Autodesk Inventor part; units mm, degrees
ref_plane "YZ Plane" through (0, 0, 0) normal (1, 0, 0) x (0, 1, 0)
ref_plane "XZ Plane" through (0, 0, 0) normal (0, 1, 0) x (-1, 0, 0)
ref_plane "XY Plane" through (0, 0, 0) normal (0, 0, 1) x (1, 0, 0)
ref_plane "Work Plane1" through (0, 0, 0) normal (0, 0, 1) x (1, 0, 0)
sketch "Sketch1" plane through (0, 0, 0) normal (0, 0, 1) x (1, 0, 0)
  circle A0 centre (132.5, -74.5) radius 1.45
  circle A1 centre (177, -74.5) radius 1.45
  line L0 (128.75, -70.75) -> (180.75, -70.75)
  line L1 (180.75, -70.75) -> (180.75, -78.25)
  line L2 (180.75, -78.25) -> (128.75, -78.25)
  line L3 (128.75, -78.25) -> (128.75, -70.75)
  circle A2 centre (132.5, -74.5) radius 1.45
  circle A3 centre (177, -74.5) radius 1.45
  point P0 (0, 0)
  dimension "d0" = 3.75
  dimension "d1" = 3.75
  dimension "d2" = 3.75
  dimension "d3" = 3.75
extrude "Extrusion1" add sketch "Sketch1" along normal blind 15
sketch "Sketch2" plane through (0, 0, 15) normal (0, 0, 1) x (1, 0, 0)
  line L0 (128.75, -78.25) -> (180.75, -78.25)
  line L1 (180.75, -78.25) -> (180.75, -70.75)
  line L2 (180.75, -70.75) -> (128.75, -70.75)
  line L3 (128.75, -70.75) -> (128.75, -78.25)
  circle A0 centre (177, -74.5) radius 1.45
  circle A1 centre (132.5, -74.5) radius 1.45
  circle A2 centre (177, -74.5) radius 1.45
  circle A3 centre (132.5, -74.5) radius 1.45
  point P0 (0, 0)
extrude "Extrusion2" add sketch "Sketch2" against normal blind 8 contours A1
sketch "Sketch4" plane through (0, 0, 15) normal (0, 0, 1) x (1, 0, 0)
  circle A0 centre (177, -74.5) radius 1.45
  circle A1 centre (177, -74.5) radius 1.45
  point P0 (0, 0)
extrude "Extrusion3" add sketch "Sketch4" against normal blind 8
sketch "Sketch5" plane through (128.75, -70.75, 0) normal (0, 1, 0) x (1, 0, 0)
  line L0 (52, 0) -> (0, 0)
  line L1 (0, 0) -> (0, -15)
  line L2 (52, -15) -> (0, -15)
  line L3 (52, 0) -> (52, -15)
  line L4 (52, -15) -> (0, -15)
  line L5 (0, -15) -> (0, 0)
  line L6 (0, 0) -> (52, 0)
  line L7 (52, 0) -> (52, -15)
  line L8 (52, -15) -> (0, -15)
  line L9 (27.805, -15) -> (30.495, -15)
  line L10 (30.495, -16) -> (27.805, -16)
  line L11 (30.495, -16) -> (30.495, -15)
  line L12 (27.805, -16) -> (27.805, -15)
  line L13 (0, -15) -> (52, -15)
  line L14 (32.545, -15) -> (52, -7.5)
  line L15 (52, 0) -> (52, -15)
  line L16 (41.9691, -6) -> (34.1871, -9) construction
  line L17 (42.5086, -7.3996) -> (34.7266, -10.3996)
  line L18 (33.6475, -7.6004) -> (41.4295, -4.6004)
  arc A0 (42.5086, -7.3996) -> (41.4295, -4.6004) centre (41.9691, -6) ccw
  arc A1 (33.6475, -7.6004) -> (34.7266, -10.3996) centre (34.1871, -9) ccw
  line L19 (20.0475, -7.6004) -> (27.8295, -4.6004)
  arc A2 (20.0475, -7.6004) -> (21.1266, -10.3996) centre (20.5871, -9) ccw
  line L20 (28.9086, -7.3996) -> (21.1266, -10.3996)
  arc A3 (28.9086, -7.3996) -> (27.8295, -4.6004) centre (28.3691, -6) ccw
  line L21 (-13.6, 0) -> (38.4, 0)
  line L22 (6.4475, -7.6004) -> (14.2295, -4.6004)
  arc A4 (6.4475, -7.6004) -> (7.5266, -10.3996) centre (6.9871, -9) ccw
  line L23 (15.3086, -7.3996) -> (7.5266, -10.3996)
  arc A5 (15.3086, -7.3996) -> (14.2295, -4.6004) centre (14.7691, -6) ccw
  line L24 (-27.2, 0) -> (24.8, 0)
  point P0 (-128.75, 0)
  point P1 (38.0781, -7.5)
  point P2 (52, -7.5)
  point P3 (32.545, -15)
  dimension "d15" = 2.05
  dimension "d21" = 6
  dimension "d22" = 6
  dimension "d23" = 1.5
  dimension "d26" = 13.6
sketch "Sketch6" plane through (0, 0, 15) normal (0, 0, 1) x (1, 0, 0)
  circle A0 centre (132.5, -74.5) radius 1.45
  line L0 (128.75, -78.25) -> (180.75, -78.25)
  line L1 (180.75, -78.25) -> (180.75, -70.75)
  line L2 (180.75, -70.75) -> (128.75, -70.75)
  line L3 (128.75, -70.75) -> (128.75, -78.25)
  circle A1 centre (132.499, -74.9265) radius 1.45
  point P0 (0, 0)
  point P1 (132.5, -74.5)
  dimension "d10" = 2.9
  dimension "d14" = 0.4265
extrude "Extrusion4" cut sketch "Sketch6" against normal blind 7 contours A1 A0 | A0 A1 picked at (132.385, -75.1117) picked at (132.6881, -76.0727)
extrude "Extrusion5" cut sketch "Sketch5" against normal blind 8 contours L3 L2 L14 | L17 A1 L18 A0 | L19 A3 L20 A2 | L22 A5 L23 A4
fillet "Fillet1" radius 1.5 3 edges at (180.75, -74.5, 7.5) (161.295, -74.5, 15) (128.75, -74.5, 15)
sketch "Sketch8" plane through (0, 0, 15) normal (0, 0, 1) x (1, 0, 0)
  circle A0 centre (157.9, -75.0575) radius 1.345
  ellipse E0 centre (158.6032, -73.9122) end of major axis (157.4109, -73.2898) minor radius 1.3427
  point P0 (0, 0)
extrude "Extrusion7" cut sketch "Sketch8" against normal blind 6.5 contours A0 E0 | A0 E0 picked at (158.3944, -74.3129) picked at (159.1018, -73.1783)
properties part number "PCB-LNA_Print_CPY"
The listing builds one solid part. Answer for the finished solid, in the listing's coordinates (mm). A direction names the side the tool comes from. Give positions to 0.01 mm unless a question says otherwise; leave off trailing zeros. Loops run counter-clockwise (first coordinate to the right, second up) from the corner with the lowest first, then second, coordinate; pieces in that order, holes last. Notation, with made-up numbers: (69.5, -30) - (124.5, -30) arc R22 cw to (124.5, -5) - close; hole circle Ø1 at (80, 73). An arc over 180 degrees is marked (long way). Return JSON: item names as keys, results as strings. Group by question number.
1. Given pin 1 Ø0.8 at (x, y) = (159, -74) entering from +Z; pin 2 Ø4.5 at (x, y) = (177, -74.5) entering from +Z; pin 3 Ø1.4 at (x, y) = (132.5, -75) entering from +Z, each flat-ended and moving along its own axis, determine where each tip first touches the part or whether it passes through.
2. Find section C-C (z = 5.75). Write down the section's boundary in (x, y).
3. Straight lines are drawn through the part: line 1 (X direction, y = -74.5, z = 3.75); line 2 (Y direction, x = 177, z = 6); line 3 (X direction, y = -75.75, z = 3.5). For each, find the intervals that lie inside material, in ascending order. Write a range as [from, to].
4. Which of the six approach directions +Z, -Z, +X, -X, +Y, -Y give full straight-line access (tool end or side, diameter ignored) to faces 5 (the cylindrical face through (133.839, -73.945, 3.451)), 6 (the flat face through (166.234, -74.448, 6.121)), 7 (the flat face through (154, -70.75, 9)), 8 (the flat face through (132, -75, 8)), 9 (the cylindrical face through (180.5, -74.6, 7.3))?
5. Find section D-D (x = 155). Write down the section's boundary in (y, z), then the cut area to 3 significant figures.
6. Find section B-B (z = 2.5). Write down the section's boundary in (x, y).
7. Find section A-A (y = -71.5). Write down the section's boundary in (x, z), then the cut area to 3 significant figures.
8. Determine the mould class of faces 1 (the cylindrical face through (178.339, -73.945, 3.451)), 2 (the cylindrical face through (147.926, -74.448, 9.509)), 3 (the flat face through (159, -74, 8.5)), 4 (the flat face through (139.034, -74.448, 6.121)) for opening direction Z: pulls with the +Z half, pulls with the -Z half, needs draft (parallel to the pull), parting line crosses it, or undercut.
Verdict:
{
 "1": {"pin 1": "stops at z = 8.5", "pin 2": "stops at z = 9.81", "pin 3": "stops at z = 8"},
 "2": {"outline": "(128.75, -78.25) - (140, -78.25) - (140, -70.75) - (128.75, -70.75) - close; (145, -78.25) - (153.6, -78.25) - (153.6, -70.75) - (145, -70.75) - close; (158.6, -78.25) - (167.2, -78.25) - (167.2, -70.75) - (158.6, -70.75) - close; (172.2, -78.25) - (180.75, -78.25) - (180.75, -70.75) - (172.2, -70.75) - close; hole circle Ø2.9 at (132.5, -74.5); hole circle Ø2.9 at (177, -74.5)"},
 "3": {"line 1": "x = [128.75, 131.05], [133.95, 175.55], [178.45, 180.75]", "line 2": "y = [-78.25, -75.95], [-73.05, -70.75]", "line 3": "x = [128.75, 131.77], [133.23, 176.27], [177.73, 180.75]"},
 "4": {"face 5": "-Z", "face 6": "+Y, -Y", "face 7": "+Z, -Z, +X, -X, +Y", "face 8": "+Z", "face 9": "+Z, +X, +Y, -Y"},
 "5": {"outline": "(-78.25, 0) - (-70.75, 0) - (-70.75, 5.21) - (-78.25, 5.21) - close; (-78.25, 8.42) - (-70.75, 8.42) - (-70.75, 15) - (-78.25, 15) - close", "area": "88.4 mm^2"},
 "6": {"outline": "(128.75, -78.25) - (180.75, -78.25) - (180.75, -70.75) - (128.75, -70.75) - close; hole circle Ø2.9 at (132.5, -74.5); hole circle Ø2.9 at (177, -74.5)"},
 "7": {"outline": "(128.75, 0) - (180.75, 0) - (180.75, 6.47) arc R1.5 ccw to (179.79, 7.87) - (161.56, 14.9) arc R1.5 ccw to (161.02, 15) - (130.25, 15) arc R1.5 ccw to (128.75, 13.5) - close; hole (135.2, 7.6) - (142.98, 4.6) arc R1.5 ccw to (144.06, 7.4) - (136.28, 10.4) arc R1.5 ccw to start; hole (148.8, 7.6) - (156.58, 4.6) arc R1.5 ccw to (157.66, 7.4) - (149.88, 10.4) arc R1.5 ccw to start; hole (162.4, 7.6) - (170.18, 4.6) arc R1.5 ccw to (171.26, 7.4) - (163.48, 10.4) arc R1.5 ccw to start", "area": "610 mm^2"},
 "8": {"face 1": "needs draft", "face 2": "undercut", "face 3": "pulls with the +Z half", "face 4": "undercut"}
}
